from build123d import *

# Parameters (mm, degrees)
LINK1_DEPTH         = 50.8
SKETCH2_R           = 50.8
BOTTOMCUT_DEPTH     = 25.4
SKETCH3_R           = 25.4
BOSS_EXTRUDE1_DEPTH = 50.8


with BuildPart() as part:
    # Sketch1 → link1 (new body)
    with BuildSketch(Plane(origin=(0, 0, 0), x_dir=(1, 0, 0), z_dir=(0, 1, 0))):
        with BuildLine():
            Line((-152.4, 76.2), (152.4, 76.2))
            ThreePointArc((152.4, 76.2), (228.6, 0), (152.4, -76.2))
            Line((152.4, -76.2), (-152.4, -76.2))
            ThreePointArc((-152.4, -76.2), (-228.6, 0), (-152.4, 76.2))
        make_face()
    extrude(amount=LINK1_DEPTH)

    # Sketch2 → bottomcut (cut)
    with BuildSketch(Plane.XZ):
        with Locations(Location((-152.4, 0, 0), (0, 0, 270))):
            Circle(SKETCH2_R)
    extrude(amount=-BOTTOMCUT_DEPTH, mode=Mode.SUBTRACT)

    # Sketch3 → Boss-Extrude1 (add)
    with BuildSketch(Plane(origin=(0, 50.8, 0), x_dir=(1, 0, 0), z_dir=(0, 1, 0))):
        with Locations(Location((152.4, 0, 0), (0, 0, 270))):
            Circle(SKETCH3_R)
    extrude(amount=BOSS_EXTRUDE1_DEPTH)


solid = part.part
Design review of the part built by this model. Coordinates are the model's own, in mm. A direction names the side the tool comes from. Round coordinates to 2 decimals unless told otherwise and drop trailing zeros. Write each loop counter-clockwise with the first axis right and the second up, starting at its lowest first coordinate (ties: lowest second). Pieces come first, ordered by that corner, then holes. Notation, with made-up numbers: (26.5, -24) - (50.5, -24) arc R24 cw to (50.5, -9) - close; hole circle Ø11 at (0.25, -26). An arc over 180 degrees is marked (long way). Use a Markdown table: item, result. Add a question column.
1. We need section D-D (y = 69). State the section outline as (x, z) points.
2. We need section C-C (x = 168.5). State the section outline as (y, z) points.
3. For faces 1 (the face through (-152, 25.4, 1)), 2 (the face through (-2, 25, -76.2)), 3 (the face through (127.604, 75.844, -5.506)), list the 3-axis set-ups (+Z, -Z, +X, -X, +Y, -Y) from which the entire face can be reached by the end or side of a thin tool; tool diameter is ignored.
4. We need section B-B (z = -44). State the section outline as (x, y) points.
5. We need section A-A (y = 19). State the section outline as (x, z) points, then the cut area to 3 significant figures.
6. Mouldability with a two-part tool opening along X and no side actions: class faces 4 (the face through (-201.992, 12.522, 11.012)), 5 (the face through (2, 25, 76.2)), 6 (the face through (-228.58, 25.04, 1.68)) as +X half, -X half, draft (parallel to the pull), parting line (faces both ways), or undercut.
7. Clearance check with flat-ended pins moving along their axes: pin 1 (2 mm diameter, centred on x = 93.5, z = -2, fed in from -Y); pin 2 (4 mm diameter, centred on x = -160, z = -18.5, fed in from -Y); pin 3 (8 mm diameter, centred on y = 74, z = -23, fed in from -X); pin 4 (10 mm diameter, centred on y = 42, z = 17.5, fed in from -X). State where each tip first meets the part, or that it passes through.
8. Wall thickness on probe 1 along X at (y, z) = (9, 0); probe 2 along Z at (x, y) = (-152, 11); probe 3 along Y at (x, z) = (199, -16.5): over which ranges is each line inside the solid? List them lowest first.
Output:
| question | item | result |
|---|---|---|
| 1 | outline | circle Ø50.8 at (152.4, 0) |
| 2 | outline | (0, -74.48) - (50.8, -74.48) - (50.8, -19.65) - (101.6, -19.65) - (101.6, 19.65) - (50.8, 19.65) - (50.8, 74.48) - (0, 74.48) - close |
| 3 | face 1 | -Y |
| 3 | face 2 | -Z, +X, -X, +Y, -Y |
| 3 | face 3 | +Y |
| 4 | outline | (-214.61, 0) - (-177.79, 0) - (-177.79, 25.4) - (-127.01, 25.4) - (-127.01, 0) - (214.61, 0) - (214.61, 50.8) - (-214.61, 50.8) - close |
| 5 | outline | (-152.4, -76.2) - (152.4, -76.2) arc R76.2 ccw to (152.4, 76.2) - (-152.4, 76.2) arc R76.2 ccw to start; hole circle Ø101.6 at (-152.4, 0) |
| 5 | area | 56,600 mm2 |
| 6 | face 4 | undercut |
| 6 | face 5 | draft |
| 6 | face 6 | -X half |
| 7 | pin 1 | stops at y = 0 |
| 7 | pin 2 | stops at y = 25.4 |
| 7 | pin 3 | stops at x = 135.54 |
| 7 | pin 4 | stops at x = -227.57 |
| 8 | probe 1 | x = -228.6 to -203.2, -101.6 to 228.6 |
| 8 | probe 2 | z = -76.2 to -50.8, 50.8 to 76.2 |
| 8 | probe 3 | y = 0 to 50.8 |
